Geometry: see drawing. Coordinates: mm, zero at the bounding-box minimum. A direction names the side the tool comes from. Give positions to 0.01 mm unless a question says otherwise; leave off trailing zeros. Write each loop counter-clockwise with the first axis right and the second up, starting at its lowest first coordinate (ties: lowest second). Pieces come first, ordered by that corner, then holes. Notation, with made-up numbers: M 79,72 L 137,72 A27 cw 137,95 Z; hole C 65,-10 d7. An arc over 180 degrees is marked long. Use a Markdown table: item, result. Add a question column.
1) Section D-D on z = 1.5. Return the cut outline in (x, y), then the cut area to 3 significant figures.
2) Pin query (flat end, axial travel): pin 1 (1.5 mm diameter, centred on x = 8.5, z = 1.5, fed in from -Y); pin 2 (1 mm diameter, centred on x = 15.5, z = 1.5, fed in from +Y). Return the tip coordinate at first contact, or that it passes through.
3) Section B-B on x = 15.5. Return the cut outline in (y, z).
4) Draft query along X for the marked faces 3, 4 and 5. Return one class per face: +X half, -X half, draft (parallel to the pull), parting line (faces both ways), or undercut.
5) Set-up query: the marked faces 1 and 2. Return all of +Z, -Z, +X, -X, +Y, -Y with unobstructed straight access to the full face (end or side cutting, diameter ignored); none if empty.
6) Line query: line 1 (Z direction, x = 15.5, y = 3.25); line 2 (X direction, y = 5.5, z = 1.2); line 3 (X direction, y = 2.25, z = 1.9). Output: solid intervals per line, ascending.
7) Section C-C on z = 2.7. Return the cut outline in (x, y).
8) Section A-A on y = 2.75. Return the cut outline in (x, z).
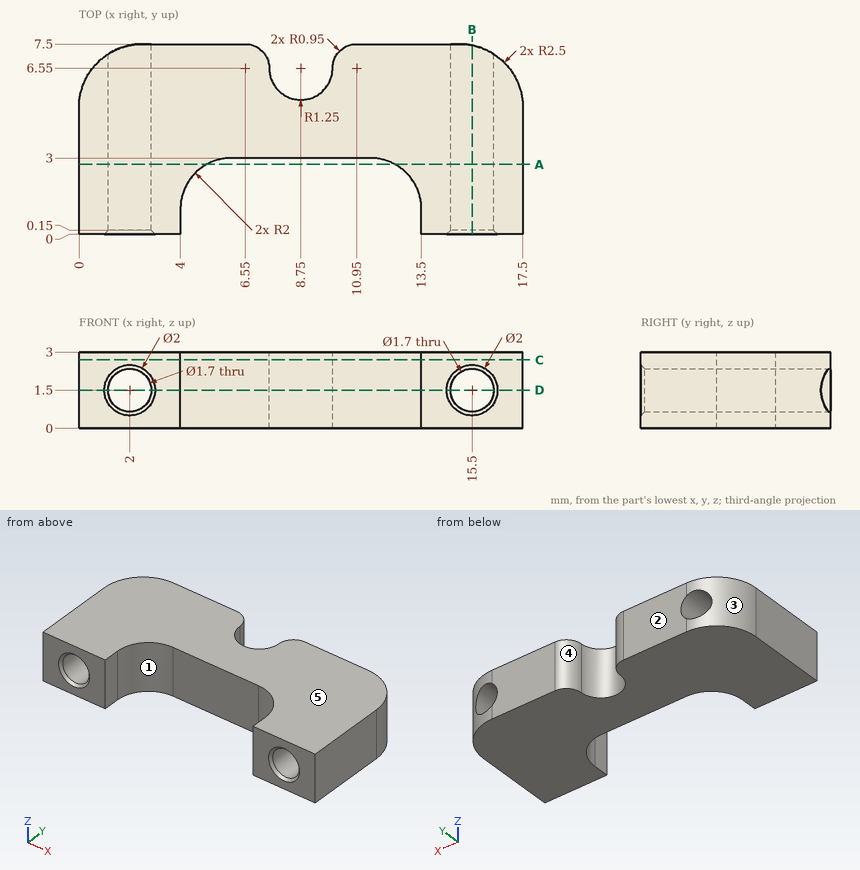
Found:
| question | item | result |
|---|---|---|
| 1 | outline | M 0,0 L 1,0 L 1.15,0.15 L 1.15,7.1 A2.5 ccw 0,5 Z; M 2.85,0.15 L 3,0 L 4,0 L 4,1 A2 cw 6,3 L 11.5,3 A2 cw 13.5,1 L 13.5,0 L 14.5,0 L 14.65,0.15 L 14.65,7.5 L 10.95,7.5 A0.95 ccw 10,6.55 A1.25 cw 7.5,6.55 A0.95 ccw 6.55,7.5 L 2.85,7.5 Z; M 16.35,0.15 L 16.5,0 L 17.5,0 L 17.5,5 A2.5 ccw 16.35,7.1 Z |
| 1 | area | 71.4 mm² |
| 2 | pin 1 | y = 3 |
| 2 | pin 2 | through |
| 3 | outline | M 0,0 L 7.45,0 L 7.45,0.65 L 0.15,0.65 L 0,0.5 Z; M 0,2.5 L 0.15,2.35 L 7.45,2.35 L 7.45,3 L 0,3 Z |
| 4 | face 3 | -X half |
| 4 | face 4 | undercut |
| 4 | face 5 | draft |
| 5 | face 1 | +Z, -Z, -Y |
| 5 | face 2 | +Z, -Z, +X, -X, +Y |
| 6 | line 1 | 0 to 0.65, 2.35 to 3 |
| 6 | line 2 | 0.05 to 1.2, 2.8 to 8.07, 9.43 to 14.7, 16.3 to 17.45 |
| 6 | line 3 | 0 to 1.25, 2.75 to 4.44, 13.06 to 14.75, 16.25 to 17.5 |
| 7 | outline | M 0,0 L 4,0 L 4,1 A2 cw 6,3 L 11.5,3 A2 cw 13.5,1 L 13.5,0 L 17.5,0 L 17.5,5 A2.5 ccw 15,7.5 L 10.95,7.5 A0.95 ccw 10,6.55 A1.25 cw 7.5,6.55 A0.95 ccw 6.55,7.5 L 2.5,7.5 A2.5 ccw 0,5 Z |
| 8 | outline | M 0,0 L 5.03,0 L 5.03,3 L 0,3 Z; M 12.47,0 L 17.5,0 L 17.5,3 L 12.47,3 Z; hole C 2,1.5 d1.7; hole C 15.5,1.5 d1.7 |
